Check sheet for the modelled part. Datum: model origin and axes. Units: mm. A direction names the side the tool comes from. Give positions to 0.01 mm unless a question says otherwise; leave off trailing zeros. Order: outer loops, then holes, each group sorted by start corner. A loop starts at its lowest first (then second) coordinate and runs counter-clockwise, first axis right, second up.
from build123d import *

# Parameters (mm, degrees)
SKETCH1_R           = 10
BOSS_EXTRUDE1_DEPTH = 5


with BuildPart() as part:
    # Sketch1 → Boss-Extrude1 (new, symmetric)
    with BuildSketch(Plane.XY):
        with BuildLine():
            ThreePointArc((-19.5, -22.79802623), (30, 0), (-19.5, 22.79802623))
            ThreePointArc((-19.5, 22.79802623), (-53.639444476, 8.591277753), (-89.625, 17.098519673))
            ThreePointArc((-89.625, 17.098519673), (-120, 0), (-89.625, -17.098519673))
            ThreePointArc((-89.625, -17.098519673), (-53.639444476, -8.591277753), (-19.5, -22.79802623))
        make_face()
        with Locations((-100, 0)):
            Circle(SKETCH1_R, mode=Mode.SUBTRACT)
        Polygon((-20, 0), (-10, -17.320508076), (10, -17.320508076), (20, 0), (10, 17.320508076), (-10, 17.320508076), align=None, mode=Mode.SUBTRACT)
    extrude(amount=BOSS_EXTRUDE1_DEPTH, both=True)


solid = part.part
1) Section check C-C, the plane x = -100. Record the cut outline in (y, z).
Recorded:
outline: (-20, -5) - (-10, -5) - (-10, 5) - (-20, 5) - close; (10, -5) - (20, -5) - (20, 5) - (10, 5) - close
2) Section check A-A, the plane x = 0. Record the cut outline in (y, z), then the cut area to 3 significant figures.
Recorded:
outline: (-30, -5) - (-17.32, -5) - (-17.32, 5) - (-30, 5) - close; (17.32, -5) - (30, -5) - (30, 5) - (17.32, 5) - close
area: 254 mm2
3) Depth check by flat-ended pin: pin 1 Ø5 at (x, z) = (-1.5, 1) entering from +Y; pin 2 Ø12 at (x, y) = (1.5, -16.5) entering from +Z; pin 3 Ø4 at (x, z) = (-57, 4) entering from -Y; pin 4 Ø4 at (y, z) = (-10, -1.5) entering from +X. Enter the tip coordinate at first touch or a pass-through.
Recorded:
pin 1: stops at y = 30
pin 2: stops at z = 5
pin 3: stops at y = -8.5
pin 4: stops at x = 28.91
4) Section check B-B, the plane z = -1.25. Record the cut outline in (x, y) (1 decimal).
Recorded:
outline: (-89.6, -17.1) arc R60 cw to (-19.5, -22.8) arc R30 ccw (long way) to (-19.5, 22.8) arc R60 cw to (-89.6, 17.1) arc R20 ccw (long way) to start; hole circle Ø20 at (-100, 0); hole (-20, 0) - (-10, -17.3) - (10, -17.3) - (20, 0) - (10, 17.3) - (-10, 17.3) - close
5) Section check D-D, the plane y = -25. Record the cut outline in (x, z).
Recorded:
outline: (-16.58, -5) - (16.58, -5) - (16.58, 5) - (-16.58, 5) - close
6) Set-up check for faces 5 (the face through (-54.16, -8.55, 0.07)), 6 (the face through (15.07, 8.54, 0.07)): record each of +Z, -Z, +X, -X, +Y, -Y from which the full face is reachable in a straight line by a thin tool's end or side.
Recorded:
face 5: +Z, -Z, -Y
face 6: +Z, -Z
7) Material ranges on L1, parallel to Y at x = -100, z = 2.25; L2, parallel to X at y = 6, z = -1.25; L3, parallel to X at y = -13, z = 4.5, recorded low to high.
Recorded:
L1: y = -20 to -10, 10 to 20
L2: x = -119.08 to -108, -92 to -16.54, 16.54 to 29.39
L3: x = -115.2 to -81.55, -35.45 to -12.49, 12.49 to 27.04
8) Draft check along X on faces 1 (the face through (29.985, -0.957, 0.07)), 2 (the face through (-53.115, 8.636, 0.07)), 3 (the face through (-46, 0, 5)), 4 (the face through (14.93, -8.78, 0.07)). Enter one of: +X half, -X half, draft (parallel to the pull), parting line (faces both ways), or undercut.
Recorded:
face 1: parting line
face 2: undercut
face 3: draft
face 4: undercut
